```python
from build123d import *

# Parameters (mm, degrees)
SKETCH_1_R      = 1
EXTRUDE_1_DEPTH = 3


with BuildPart() as part:
    # 草图1 → 凸台-拉伸1 (new body)
    with BuildSketch(Plane.XY):
        with BuildLine():
            Line((5, 0), (5, -2.598546895))
            ThreePointArc((5, -2.598546895), (4.894337932, -3.387728708), (4.584794711, -4.121319466))
            Line((4.584794711, -4.121319466), (3.415205289, -6.106611695))
            ThreePointArc((3.415205289, -6.106611695), (3.105662068, -6.840202453), (3, -7.629384266))
            Line((3, -7.629384266), (3, -32.42729606))
            Line((3, -32.42729606), (3.807110108, -36.292324141))
            Line((3.807110108, -36.292324141), (5.41514713, -39.807586397))
            Line((5.41514713, -39.807586397), (8.899761864, -45.72298083))
            Line((8.899761864, -45.72298083), (9.562607856, -46.702581702))
            Line((9.562607856, -46.702581702), (7.077963413, -48.383813985))
            Line((7.077963413, -48.383813985), (6.565734565, -47.626805824))
            Line((6.565734565, -47.626805824), (0.880089764, -37.974998041))
            ThreePointArc((0.880089764, -37.974998041), (0.834425065, -37.894675513), (0.79125555, -37.812984837))
            Line((0.79125555, -37.812984837), (-1.794096527, -32.732789057))
            ThreePointArc((-1.794096527, -32.732789057), (-1.927277743, -32.438160812), (-2.032701862, -32.132499572))
            Line((-2.032701862, -32.132499572), (-4.857906932, -22.522211807))
            ThreePointArc((-4.857906932, -22.522211807), (-4.964294608, -22.033724953), (-5, -21.535063876))
            Line((-5, -21.535063876), (-5, 0))
            ThreePointArc((-5, 0), (0, 5), (5, 0))
        make_face()
        with Locations((0, -15)):
            Circle(SKETCH_1_R, mode=Mode.SUBTRACT)
        with BuildLine():
            Line((-3, -25), (-3, 0))
            ThreePointArc((-3, 0), (2.323790008, 1.897366596), (-0.6, -2.939387691))
            ThreePointArc((-0.6, -2.939387691), (-1.432455532, -3.144586919), (-1.8, -3.919183588))
            Line((-1.8, -3.919183588), (-1.8, -25))
            ThreePointArc((-1.8, -25), (-2.4, -25.6), (-3, -25))
        make_face(mode=Mode.SUBTRACT)
    extrude(amount=EXTRUDE_1_DEPTH)


solid = part.part
```
Read the model definition and answer for the solid it produces. Units are mm, in the model's axes. A direction names the side the tool comes from. Round coordinates to 2 decimals unless told otherwise and drop trailing zeros. Write each loop counter-clockwise with the first axis right and the second up, starting at its lowest first coordinate (ties: lowest second). Pieces come first, ordered by that corner, then holes. Notation, with made-up numbers: (43, 54) - (48, 54) arc R22 ccw to (48, 81) - close; hole circle Ø7 at (64, 50). An arc over 180 degrees is marked (long way). One line per item, written item: value.
Q1. Find section C-C (z = 2). Count the separate pieces of the cut face and the enclosed holes in it, and give its area (3 significant figures).
The answers:
separate pieces: 1
enclosed holes: 2
area: 289 mm2
Q2. Find section D-D (y = -29). Determine the outline of the cut face in (x, z), and give its area (3 significant figures).
The answers:
outline: (-2.95, 0) - (3, 0) - (3, 3) - (-2.95, 3) - close
area: 17.9 mm2
Q3. Find section B-B (x = 0). Determine the outline of the cut face in (y, z).
The answers:
outline: (-36.26, 0) - (-16, 0) - (-16, 3) - (-36.26, 3) - close; (-14, 0) - (-3, 0) - (-3, 3) - (-14, 3) - close; (3, 0) - (5, 0) - (5, 3) - (3, 3) - close
Q4. Each of these flat-tipped pins is pushed along its axis until it touches: P1, Ø1, axis at y = -18, z = 2, coming from the +X side; P2, Ø1.5, axis at y = -4.5, z = 0.5, coming from the +X side. Where does it stop, or does it pass through?
The answers:
P1: stops at x = 3
P2: stops at x = 4.77
Q5. Straight lines are drawn through the part: line 1 (Y direction, x = -0.25, z = 0.55); line 2 (Y direction, x = 0, z = 1); line 3 (X direction, y = -10, z = 1.85). For each, find the intervals that lie inside material, in ascending order. Write a range as from..to.
The answers:
line 1: y = -35.77..-15.97, -14.03..-2.99, 2.99..4.99
line 2: y = -36.26..-16, -14..-3, 3..5
line 3: x = -5..-3, -1.8..3
Q6. Find section A-A (y = -9). Determine the outline of the cut face in (x, z), and give its area (3 significant figures).
The answers:
outline: (-5, 0) - (-3, 0) - (-3, 3) - (-5, 3) - close; (-1.8, 0) - (3, 0) - (3, 3) - (-1.8, 3) - close
area: 20.4 mm2
Q7. Which of the six approach directions +Z, -Z, +X, -X, +Y, -Y give full straight-line access (tool end or side, diameter ignored) to faces 4 (the flat face through (9.23, -46.21, 1.48)), 5 (the cylindrical face through (3.11, -6.83, 1.48)), 6 (the cylindrical face through (-1.423, -3.137, 1.479))?
The answers:
face 4: +Z, -Z, +X, +Y
face 5: +Z, -Z, +X
face 6: +Z, -Z
Q8. For a pull along Y with two mould halves and no side action, classify faces 1 (the flat face through (4.01, -5.1, 1.48)), 2 (the flat face through (-3.426, -27.395, 1.479)), 3 (the flat face through (5, -1, 1)) as pulls with the +Y half, pulls with the -Y half, needs draft (parallel to the pull), parting line crosses it, or undercut.
The answers:
face 1: undercut
face 2: pulls with the -Y half
face 3: needs draft
